Geometry check sheet. Reference: the model listing, model coordinates, mm. Give positions to 0.01 mm unless a question says otherwise; leave off trailing zeros. Loops run counter-clockwise (first coordinate to the right, second up) from the corner with the lowest first, then second, coordinate; pieces in that order, holes last.
1. Cross-section at B-B, the plane y = 2.1. State how many separate pieces and enclosed holes the cut face has, plus the area to 3 significant figures.
2. Cross-section at C-C, the plane z = -13.5. Record the cut outline in (x, y) (3 decimals).
3. Material ranges on L1, parallel to Z at x = 0, y = 1.1; L2, parallel to X at y = 0.6, z = 60; L3, parallel to Z at x = 2, y = 2, recorded low to high.
4. Cross-section at A-A, the plane z = -25.4. Record the cut outline in (x, y), plus the area to 3 significant figures.
5. Go/stop test with flat-tipped pins: pin 1 Ø3.5 at (x, z) = (0, 76.2) entering from +Y; pin 2 Ø8 at (x, z) = (50.8, 50.8) entering from -Y; pin 3 Ø0.8 at (y, z) = (0.5, 27) entering from -X. Record where each tip stops, or that it passes through.
from build123d import *

# Parameters (mm, degrees)
BOSS_EXTRUDE2_DEPTH = 3
BOSS_EXTRUDE3_DEPTH = 1.5
SKETCH4_R           = 3
CUT_EXTRUDE1_DEPTH  = 10
CIRPATTERN2_COUNT   = 7
CIRPATTERN2_ANGLE   = 90
SKETCH7_R           = 3.047588699
BOSS_EXTRUDE5_DEPTH = 3
SKETCH7_3_R         = 3.047588699
CUT_EXTRUDE2_DEPTH  = 3
FILLET1_R           = 6


with BuildPart() as part:
    # Sketch2 → Boss-Extrude2 (new body)
    with BuildSketch(Plane(origin=(0, 0, 0), x_dir=(1, 0, 0), z_dir=(0, 1, 0))):
        with BuildLine():
            ThreePointArc((32.5, 0), (19.784746443, -25.783983559), (-8.411618966, -31.392589354))
            Line((-8.411618966, -31.392589354), (-19.411428383, -72.444436972))
            ThreePointArc((-19.411428383, -72.444436972), (45.657107176, -59.501500522), (75, 0))
            ThreePointArc((75, 0), (74.358364603, 9.789464417), (72.444436972, 19.411428383))
            Line((72.444436972, 19.411428383), (31.392589354, 8.411618966))
            ThreePointArc((31.392589354, 8.411618966), (32.221957995, 4.242101247), (32.5, 0))
        make_face()
    extrude(amount=BOSS_EXTRUDE2_DEPTH)

    # Sketch3 → Boss-Extrude3 (add)
    with BuildSketch(Plane.XZ):
        with BuildLine():
            ThreePointArc((8.411618966, 31.392589354), (0, 32.5), (-8.411618966, 31.392589354))
            Line((-8.411618966, 31.392589354), (8.411618966, 31.392589354))
        make_face()
        with BuildLine():
            Line((28.494811876, -7.635161831), (31.392589354, -8.411618966))
            ThreePointArc((31.392589354, -8.411618966), (32.221957995, -4.242101247), (32.5, 0))
            ThreePointArc((32.5, 0), (27.378025192, 17.512673599), (13.626539288, 29.505379629))
            Line((13.626539288, 29.505379629), (13.626539288, 26.16423947))
            ThreePointArc((13.626539288, 26.16423947), (25.221349181, 15.30142299), (29.5, 0))
            ThreePointArc((29.5, 0), (29.247623411, -3.85052267), (28.494811876, -7.635161831))
        make_face()
    extrude(amount=-BOSS_EXTRUDE3_DEPTH)

    # Sketch4 → Cut-Extrude1 (cut)
    with BuildSketch(Plane(origin=(0, 3, 0), x_dir=(1, 0, 0), z_dir=(0, 1, 0))):
        with Locations((0, -42.5)):
            Circle(SKETCH4_R)
        with Locations((0, -52.5)):
            Circle(SKETCH4_R)
        with Locations((0, -62.5)):
            Circle(SKETCH4_R)
    cut_extrude1 = extrude(amount=-CUT_EXTRUDE1_DEPTH, mode=Mode.SUBTRACT)

    # CirPattern2: Cut-Extrude1 ×7 about axis
    cirpattern2_axis = Axis((0, 0, 0), (0, 1, 0))
    for i in range(1, CIRPATTERN2_COUNT):
        add(cut_extrude1.rotate(cirpattern2_axis, i * CIRPATTERN2_ANGLE / (CIRPATTERN2_COUNT - 1)), mode=Mode.SUBTRACT)

    # Sketch7 → Boss-Extrude5 (add)
    with BuildSketch(Plane.XZ):
        with BuildLine():
            Line((-5.404581923, 76.2), (-19.411428383, 72.444436972))
            ThreePointArc((-19.411428383, 72.444436972), (-11.165518609, 74.164217748), (-2.77876912, 74.94850527))
            ThreePointArc((-2.77876912, 74.94850527), (0, 79.247588699), (2.77876912, 74.94850527))
            ThreePointArc((2.77876912, 74.94850527), (9.318606025, 74.41883889), (15.78712451, 73.319620155))
            Line((15.78712451, 73.319620155), (5.404581923, 76.2))
            ThreePointArc((5.404581923, 76.2), (0, 81.604581923), (-5.404581923, 76.2))
        make_face()
        with BuildLine():
            ThreePointArc((49.770964897, 56.105713196), (53.033008589, 53.033008589), (56.105713196, 49.770964897))
            ThreePointArc((56.105713196, 49.770964897), (54.621616527, 54.621616527), (49.770964897, 56.105713196))
        make_face()
        with BuildLine():
            Line((50.264676908, -9.974138925), (45.819583471, -23.301201068))
            ThreePointArc((45.819583471, -23.301201068), (49.037057403, -30.508966545), (56.0148967, -26.819280865))
            Line((56.0148967, -26.819280865), (58.942789983, -15.793672976))
            Line((58.942789983, -15.793672976), (58.942789983, -12.868627078))
            Line((58.942789983, -12.868627078), (50.264676908, -9.974138925))
        make_face()
        with Locations((50.8, -25.4)):
            Circle(SKETCH7_R, mode=Mode.SUBTRACT)
    extrude(amount=-BOSS_EXTRUDE5_DEPTH)

    # Sketch7<3> → Cut-Extrude2 (cut)
    with BuildSketch(Plane.XZ):
        with Locations((0, 76.2)):
            Circle(SKETCH7_3_R)
        with Locations((50.8, 50.8)):
            Circle(SKETCH7_3_R)
    extrude(amount=-CUT_EXTRUDE2_DEPTH, mode=Mode.SUBTRACT)

    # Fillet1
    fillet1_edges = [part.edges().sort_by_distance(p)[0] for p in [
        (49.194825936, 1.5, -13.181713881),
        (58.942789983, 1.5, -15.793672976),
    ]]
    fillet(fillet1_edges, radius=FILLET1_R)


solid = part.part
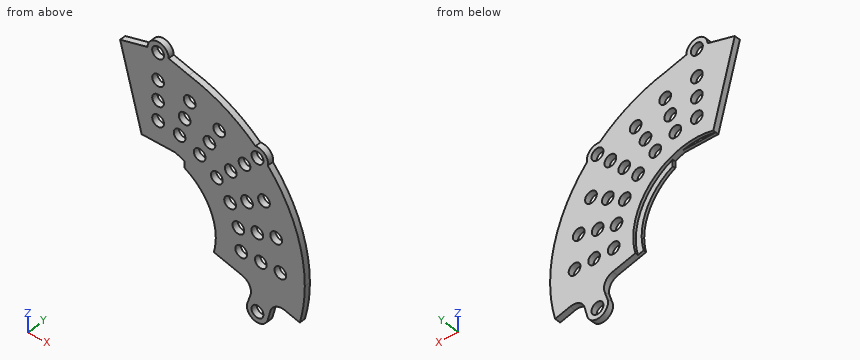
Result:
1. separate pieces: 1
1. enclosed holes: 24
1. area: 4,370 mm2
2. outline: (46.107, 0) - (73.775, 0) - (73.775, 3) - (46.107, 3) - close
3. L1: z = 31.39 to 39.5, 45.5 to 49.5, 55.5 to 59.5, 65.5 to 73.15, 79.25 to 81.6
3. L2: x = -16.08 to -1.66, 1.66 to 13.2, 19.15 to 45
3. L3: z = 32.44 to 40.26, 44.74 to 50.26, 54.74 to 60.26, 64.74 to 73.9, 78.5 to 81.22
4. outline: (45.4, 0) - (47.75, 0) - (47.75, 3) - (45.4, 3) - close; (53.85, 0) - (56.39, 0) - (56.39, 3) - (53.85, 3) - close
4. area: 14.7 mm2
5. pin 1: passes through
5. pin 2: stops at y = 0
5. pin 3: stops at x = 13.63
